Autodesk Inventor part; units mm, degrees
ref_plane "YZ Plane" through (0, 0, 0) normal (1, 0, 0) x (0, 1, 0)
ref_plane "XZ Plane" through (0, 0, 0) normal (0, 1, 0) x (-1, 0, 0)
ref_plane "XY Plane" through (0, 0, 0) normal (0, 0, 1) x (1, 0, 0)
sketch "Sketch1" plane through (0, 0, 0) normal (1, 0, 0) x (0, 1, 0)
  circle A0 centre (0, 0) radius 4.445
  circle A1 centre (0, 0) radius 8.255
  dimension "d0" = 8.89
  dimension "d1" = 3.81
extrude "Extrusion1" add sketch "Sketch1" along normal blind 19.812
sketch "Sketch2" plane through (0, 0, 0) normal (-1, 0, 0) x (0, 0, 1)
  circle A0 centre (0, 0) radius 8.255
  circle A1 centre (0, 0) radius 7.747
  circle A2 centre (0, 0) radius 8.255
  dimension "d42" = 0
extrude "Extrusion2" add sketch "Sketch2" along normal blind 2.54 contours A0 | A1
sketch "Sketch3" plane through (-2.54, 0, 0) normal (-1, 0, 0) x (0, 0, 1)
  line L0 (19.05, 48.5955) -> (-19.05, 48.5955)
  circle A0 centre (0, 0) radius 8.255
  line L1 (8.255, 0) -> (19.05, 48.5955)
  line L2 (-8.255, 0) -> (-19.05, 48.5955)
  arc A1 (8.255, 0) -> (-8.255, 0) centre (0, 0) ccw
  line L3 (-14.3008, 44.7855) -> (14.3008, 44.7855)
  line L4 (14.3008, 44.7855) -> (6.5962, 10.1022)
  arc A2 (6.5962, 10.1022) -> (-6.5962, 10.1022) centre (0, 0) ccw
  line L5 (-6.5962, 10.1022) -> (-14.3008, 44.7855)
  dimension "d6" = 38.1
  dimension "d7" = 19.05
  dimension "d8" = 3.81
extrude "Extrusion3" add sketch "Sketch3" against normal blind 6.35 contours L1 A0 L2 L0
sketch "Sketch6" plane through (-2.54, 44.7855, -14.3008) normal (0, -1, 0) x (1, 0, 0)
  line L0 (6.35, 32.4159) -> (26.9875, 32.4159)
  line L1 (13.4874, 32.4159) -> (13.4874, 26.0989)
  line L2 (26.9875, 32.4159) -> (26.9875, -3.9117)
  point P0 (2.54, 14.3008)
  dimension "d20" = 13.5001
sketch "Sketch10" plane through (0, 0, 0) normal (1, 0, 0) x (0, 0, -1)
  circle A0 centre (0, 0) radius 1.4542
  line L0 (-4.445, 1.4542) -> (4.445, 1.4542)
  line L1 (4.445, 1.4542) -> (4.445, -1.4542)
  line L2 (4.445, -1.4542) -> (-4.445, -1.4542)
  line L3 (-4.445, -1.4542) -> (-4.445, 1.4542)
  circle A1 centre (0, 0) radius 4.445
  dimension "d43" = 0
  dimension "d44" = 0
extrude "Extrusion7" cut sketch "Sketch10" against normal blind 22.225 contours A0 | A0 L0 A1 L2 | A0 L2 A1 L0 | A1 L3 L0 | L0 L1 A1 | A1 L1 L2 | L2 L3 A1
sketch "Sketch14" plane through (0, 0, 0) normal (-1, 0, 0) x (0, 0, 1)
  arc A0 (4.2004, -1.4542) -> (4.445, 0) centre (0, 0) ccw
  line L0 (4.2004, -1.4542) -> (4.445, -1.4542)
  line L1 (4.445, -1.4542) -> (4.445, 0)
  arc A1 (4.445, 0) -> (4.2004, 1.4542) centre (0, 0) ccw
  line L2 (4.445, 0) -> (4.445, 1.4542)
  line L3 (4.445, 1.4542) -> (4.2004, 1.4542)
  arc A2 (-4.445, 0) -> (-4.2004, -1.4542) centre (0, 0) ccw
  line L4 (-4.445, 0) -> (-4.445, -1.4542)
  line L5 (-4.445, -1.4542) -> (-4.2004, -1.4542)
  arc A3 (-4.2004, 1.4542) -> (-4.445, 0) centre (0, 0) ccw
  line L6 (-4.2004, 1.4542) -> (-4.445, 1.4542)
  line L7 (-4.445, 1.4542) -> (-4.445, 0)
extrude "Extrusion10" add sketch "Sketch14" along normal blind 2.54
sketch "Sketch15" plane through (-2.54, 0, 0) normal (-1, 0, 0) x (0, 0, 1)
  circle A0 centre (0, 0) radius 41.275
  circle A1 centre (0, 0) radius 44.45
  dimension "d47" = 82.55
  dimension "d48" = 88.9
extrude "Extrusion11" add sketch "Sketch15" against normal blind 2.54
sketch "Sketch16" plane through (0, 0, 0) normal (1, 0, 0) x (0, 0, -1)
  circle A0 centre (0, 0) radius 44.45
  circle A1 centre (0, 0) radius 41.275
  dimension "d51" = 82.55
extrude "Extrusion12" add sketch "Sketch16" along normal blind 38.1
sketch "Sketch19" plane through (-2.54, 0, 0) normal (-1, 0, 0) x (0, 0, 1)
  line L0 (4.2004, 1.4542) -> (-4.2004, 1.4542)
  arc A0 (-16.6452, 37.7699) -> (16.6452, 37.7699) centre (0, 0) ccw
  line L1 (-4.2004, 1.4542) -> (-41.2494, 1.4542)
  line L2 (4.2004, 1.4542) -> (41.2494, 1.4542)
  circle A1 centre (0, 0) radius 8.382
  line L3 (-4.2004, -1.4542) -> (4.2004, -1.4542)
  line L4 (4.2004, 1.4542) -> (-4.2004, 1.4542)
  line L5 (-41.2494, -1.4542) -> (41.2494, -1.4542)
extrude "Extrusion14" add sketch "Sketch19" against normal blind 6.35 contours L2 A1 L5 L3 L1 L0 | L2 A0 L5 A1 | A1 L5 A0 L1
sketch "Sketch20" plane through (3.81, 0, 0) normal (1, 0, 0) x (0, 0, -1)
  arc A0 (4.2004, -1.4542) -> (4.2004, 1.4542) centre (0, 0) ccw
  line L0 (4.2004, 1.4542) -> (-4.2004, 1.4542)
  arc A1 (-4.2004, 1.4542) -> (-4.2004, -1.4542) centre (0, 0) ccw
  line L1 (-4.2004, -1.4542) -> (4.2004, -1.4542)
extrude "Extrusion15" cut sketch "Sketch20" against normal blind 6.35
sketch "Sketch21" plane through (-2.54, 0, 0) normal (-1, 0, 0) x (0, 0, 1)
  arc A0 (-8.1259, -1.4542) -> (8.1259, -1.4542) centre (0, 0) ccw
  line L0 (1.8212, -8.0516) -> (1.8212, -41.2348)
  arc A1 (-41.2494, -1.4542) -> (41.2494, -1.4542) centre (0, 0) ccw
  line L1 (-1.8492, -41.2336) -> (-1.8492, -8.1755)
  arc A2 (-1.8492, -41.2336) -> (1.8212, -41.2348) centre (0, 0) ccw
  circle A3 centre (0, 0) radius 8.255
  arc A4 (-1.8492, -8.0452) -> (1.8212, -8.0516) centre (0, 0) ccw
  line L2 (-1.8492, -8.1755) -> (-1.8492, -8.0452)
extrude "Extrusion16" add sketch "Sketch21" against normal blind 6.35 contours A0 L0 A1 L1 L2
sketch "Sketch24" plane through (38.1, 0, 0) normal (1, 0, 0) x (0, 0, -1)
  circle A0 centre (0, 0) radius 53.866
  circle A1 centre (0, 0) radius 44.45
extrude "Extrusion18" cut sketch "Sketch24" against normal blind 61.9125
properties part number "Lift motor v2[FINAL]"
Source: CAD feature listing. Evaluate the final solid. Frame: model axes, mm. A direction names the side the tool comes from. Coordinates: 2 decimals unless noted, no trailing zeros. Loops run counter-clockwise (first coordinate to the right, second up) from the corner with the lowest first, then second, coordinate; pieces in that order, holes last. Notation, with made-up numbers: M 65,86 L 92,86 A26 cw 92,113 Z; hole C 52.25,3 d8. An arc over 180 degrees is marked long. Answer in a Markdown table with one row per item.
Q1. Draft query along Y for faces 4 (the flat face through (-1, -1.454, 0)), 5 (the flat face through (-2.54, -3, 0)), 6 (the cylindrical face through (17.496, 40.293, 8.948)). Return one class per face: pulls with the +Y half, pulls with the -Y half, needs draft (parallel to the pull), parting line crosses it, or undercut.
Answers below:
| item | result |
|---|---|
| face 4 | undercut |
| face 5 | needs draft |
| face 6 | undercut |
Q2. Section D-D on x = 8. Return the cut outline in (y, z) (3 decimals), plus the area to 3 significant figures.
Answers below:
| item | result |
|---|---|
| outline | C 0,0 d88.9; C 0,0 d16.51; hole C 0,0 d82.55; hole C 0,0 d8.89 |
| area | 1,010 mm^2 |
Q3. Set-up query: faces 1 (the cylindrical face through (10.963, -6.551, 5.023)), 2 (the flat face through (-1, 1.454, 0)), 3 (the flat face through (38.1, -29.4, -29.4)). Return all of +Z, -Z, +X, -X, +Y, -Y with unobstructed straight access to the full face (end or side cutting, diameter ignored); none if empty.
Answers below:
| item | result |
|---|---|
| face 1 | +X |
| face 2 | +X, -X |
| face 3 | +Z, -Z, +X, +Y, -Y |
Q4. Section C-C on y = -6. Return the cut outline in (x, z).
Answers below:
| item | result |
|---|---|
| outline | M -2.54,-44.04 L 38.1,-44.04 L 38.1,-40.84 L -2.54,-40.84 Z; M -2.54,-5.67 L 19.81,-5.67 L 19.81,5.67 L -2.54,5.67 Z; M -2.54,40.84 L 38.1,40.84 L 38.1,44.04 L -2.54,44.04 Z |
Q5. First-contact query: pin 1 (3 mm diameter, centred on x = 1, z = -19.5, fed in from -Y); pin 2 (1.5 mm diameter, centred on x = 9, y = -2.5, fed in from +Z); pin 3 (1.9 mm diameter, centred on x = -0.5, z = 20.5, fed in from -Y). Flat tips, straight axial feed; report the tip coordinate or a pass-through.
Answers below:
| item | result |
|---|---|
| pin 1 | stops at y = -40.64 |
| pin 2 | stops at z = 44.42 |
| pin 3 | stops at y = -39.92 |
Q6. Ray query, probe 1 along Y at (x, z) = (14.75, 0) (3 decimals); probe 2 along Y at (x, z) = (2.5, -1). Return the intervals inside material, ascending. Write a range as from..to.
Answers below:
| item | result |
|---|---|
| probe 1 | y = -44.45..-41.275, -8.255..-4.445, 4.445..8.255, 41.275..44.45 |
| probe 2 | y = -44.44..-4.33, 4.33..12.02, 41.26..44.44 |
Q7. Section B-B on z = -23. Return the cut outline in (x, y).
Answers below:
| item | result |
|---|---|
| outline | M -2.54,-38.04 L 38.1,-38.04 L 38.1,-34.27 L -2.54,-34.27 Z; M -2.54,-1.45 L 3.81,-1.45 L 3.81,1.45 L -2.54,1.45 Z; M -2.54,34.27 L 38.1,34.27 L 38.1,38.04 L -2.54,38.04 Z |
